Autodesk Inventor part; units mm, degrees
ref_plane "YZ Plane" through (0, 0, 0) normal (1, 0, 0) x (0, 1, 0)
ref_plane "XZ Plane" through (0, 0, 0) normal (0, 1, 0) x (-1, 0, 0)
ref_plane "XY Plane" through (0, 0, 0) normal (0, 0, 1) x (1, 0, 0)
sketch "Boceto1" plane through (0, 0, 0) normal (0, 1, 0) x (-1, 0, 0)
  line L0 (7.1, 11.7) -> (-7.1, 11.7)
  line L1 (-7.1, 11.7) -> (-7.1, -11.7)
  line L2 (-7.1, -11.7) -> (7.1, -11.7)
  line L3 (7.1, -11.7) -> (7.1, 11.7)
  line L4 (7.1, 11.7) -> (-7.1, -11.7) construction
  line L5 (-7.1, 11.7) -> (7.1, -11.7) construction
  circle A0 centre (4.1, 7.85) radius 1.45
  circle A1 centre (-4.1, 7.85) radius 1.45
  circle A2 centre (4.1, -7.85) radius 1.45
  circle A3 centre (-4.1, -7.85) radius 1.45
  point P0 (0, 0)
  dimension "d0" = 23.4
  dimension "d1" = 14.2
  dimension "d2" = 2.9
  dimension "d3" = 8.2
  dimension "d4" = 4.1
  dimension "d5" = 7.85
  dimension "d6" = 7.85
extrude "Extrusión1" add sketch "Boceto1" along normal blind 2
sketch "Boceto2" plane through (0, 2, 0) normal (0, 1, 0) x (1, 0, 0)
  line L0 (-7.1, 11.7) -> (-7.1, -11.7)
  line L1 (7.1, -3.775) -> (-7.1, -3.775)
  line L2 (-7.1, -3.775) -> (-7.1, 3.775)
  line L3 (-7.1, 3.775) -> (7.1, 3.775)
  line L4 (7.1, 3.775) -> (7.1, -3.775)
  line L5 (7.1, -3.775) -> (-7.1, 3.775) construction
  line L6 (-7.1, -3.775) -> (7.1, 3.775) construction
  point P0 (0, 0)
  point P1 (-7.1, 9.7)
  point P2 (-7.1, -9.7)
  point P3 (-7.1, -3.775)
  dimension "d10" = 7.55
extrude "Extrusión2" add sketch "Boceto2" along normal blind 2
sketch "Boceto3" plane through (0, 0, 0) normal (0, -1, 0) x (1, 0, 0)
  line L0 (-7.1, 11.7) -> (7.1, 11.7)
  line L1 (-7.1, -11.7) -> (-7.1, 11.7)
  line L2 (7.1, -11.7) -> (-7.1, -11.7)
  line L3 (7.1, 11.7) -> (7.1, -11.7)
  circle A0 centre (-4.1, 7.85) radius 1.45
  circle A1 centre (4.1, 7.85) radius 1.45
  circle A2 centre (-4.1, -7.85) radius 1.45
  circle A3 centre (4.1, -7.85) radius 1.45
  point P0 (0, 0)
extrude "Extrusión3" add sketch "Boceto3" along normal blind 14
sketch "Boceto5" plane through (0, -14, 0) normal (0, -1, 0) x (1, 0, 0)
  line L0 (7.1, -11.7) -> (7.1, 11.7)
  line L1 (-7.1, -6) -> (7.1, -6)
  line L2 (7.1, -6) -> (7.1, 6)
  line L3 (7.1, 6) -> (-7.1, 6)
  line L4 (-7.1, 6) -> (-7.1, -6)
  line L5 (-7.1, -6) -> (7.1, 6) construction
  line L6 (7.1, -6) -> (-7.1, 6) construction
  point P0 (0, 0)
  point P1 (7.1, -9.7)
  point P2 (7.1, 9.7)
  point P3 (7.1, -6)
  dimension "d16" = 12
extrude "Extrusión4" add sketch "Boceto5" along normal blind 14
sketch "Boceto7" plane through (0, -14, 0) normal (0, -1, 0) x (1, 0, 0)
  circle A0 centre (-4.1, 7.85) radius 1.45
  circle A1 centre (4.1, 7.85) radius 1.45
  circle A2 centre (4.1, -7.85) radius 1.45
  circle A3 centre (-4.1, -7.85) radius 1.45
  point P0 (0, 0)
extrude "Extrusión6" add sketch "Boceto7" against normal blind 0.5
fillet "Empalme3" radius 8 2 edges at (0, -14, 6) (0, -14, -6)
fillet "Empalme4" radius 7 2 edges at (0, -28, -6) (0, -28, 6)
fillet "Empalme5" radius 7 2 edges at (0, -14, -11.7) (0, -14, 11.7)
sketch "Boceto8" plane through (-7.1, 2, 3.775) normal (-1, 0, 0) x (0, 0, 1)
  arc A0 (-10.3083, -20.7902) -> (2.7583, -20.7902) centre (-3.775, -18.2771) ccw
  circle A1 centre (-3.775, -18.2771) radius 5.075
  point P0 (-3.775, -2)
  dimension "d28" = 10.15
extrude "Extrusión7" cut sketch "Boceto8" against normal through all
properties part number "MiddleJoint"
Source: CAD feature listing. Evaluate the final solid. Frame: model axes, mm. A direction names the side the tool comes from. Round coordinates to 2 decimals unless told otherwise and drop trailing zeros. Write each loop counter-clockwise with the first axis right and the second up, starting at its lowest first coordinate (ties: lowest second). Pieces come first, ordered by that corner, then holes. Notation, with made-up numbers: M 3.25,0 L 58.25,0 A13 ccw 58.25,21 Z; hole C 60,-38 d5. An arc over 180 degrees is marked long. One line per item, written item: value. Start each with the question number.
Item 1: Set-up query: faces 1 (the cylindrical face through (-0.1, -12.9, -11.02)), 2 (the flat face through (0, 3, 3.775)), 3 (the flat face through (0, 2, -8)), 4 (the flat face through (-4, -13.5, -8)), 5 (the cylindrical face through (0.1, -16.94, 7.54)). Return all of +Z, -Z, +X, -X, +Y, -Y with unobstructed straight access to the full face (end or side cutting, diameter ignored); none if empty.
Item 2: Section query C-C (z = -7.85). Return the cut outline in (x, y), plus the area to 3 significant figures.
Item 3: Section query A-A (y = -12.75). Return the cut outline in (x, z).
Item 4: Ray query, L1, parallel to X at y = 0.5, z = 8; L2, parallel to Z at x = 4.1, y = 0.65; L3, parallel to Z at x = -5.25, y = -4.25. Return the intervals inside material, ascending. Write a range as from..to.
Item 5: Section query D-D (y = -18). Return the cut outline in (x, z).
Item 6: Section query B-B (y = 1). Return the cut outline in (x, z), plus the area to 3 significant figures.
Item 7: Mould query, pull axis X, two halves, no side actions, for faces 6 (the flat face through (4, -13.5, -8)), 7 (the flat face through (0, -4, -11.7)), 8 (the flat face through (-7.1, -6, 0)). Classes: pulls with the +X half, pulls with the -X half, needs draft (parallel to the pull), parting line crosses it, or undercut.
Item 8: Pin query (flat end, axial travel): pin 1 (8.5 mm diameter, centred on x = 0.5, z = -6, fed in from +Y); pin 2 (2.5 mm diameter, centred on x = 4.1, z = -7.85, fed in from -Y); pin 3 (2.5 mm diameter, centred on x = -4.5, z = -7.5, fed in from +Y); pin 4 (3 mm diameter, centred on x = -3.5, z = 2, fed in from -Y). Return the tip coordinate at first contact, or that it passes through.
Result set:
1. face 1: -Z, +X, -X, -Y
1. face 2: +Z, +X, -X, +Y
1. face 3: -Z, +X, -X, +Y
1. face 4: +Y
1. face 5: +Z, +X, -X, -Y
2. outline: M -7.1,-16.55 L 7.1,-16.55 L 7.1,2 L 5.55,2 L 5.55,-13.5 L 2.65,-13.5 L 2.65,2 L -2.65,2 L -2.65,-13.5 L -5.55,-13.5 L -5.55,2 L -7.1,2 Z
2. area: 173 mm²
3. outline: M -7.1,-11.09 L 7.1,-11.09 L 7.1,-3.65 L -7.1,-3.65 Z; M -7.1,3.65 L 7.1,3.65 L 7.1,11.09 L -7.1,11.09 Z; hole C -4.1,-7.85 d2.9; hole C -4.1,7.85 d2.9; hole C 4.1,-7.85 d2.9; hole C 4.1,7.85 d2.9
4. L1: x = -7.1..-5.54, -2.66..2.66, 5.54..7.1
4. L2: z = -11.7..-9.3, -6.4..6.4, 9.3..11.7
4. L3: z = -11.7..-8.73, -6.97..6.97, 8.73..11.7
5. outline: M -7.1,-6.89 L 7.1,-6.89 L 7.1,-4.77 L -7.1,-4.77 Z; M -7.1,4.77 L 7.1,4.77 L 7.1,6.89 L -7.1,6.89 Z
6. outline: M -7.1,-11.7 L 7.1,-11.7 L 7.1,11.7 L -7.1,11.7 Z; hole C -4.1,-7.85 d2.9; hole C -4.1,7.85 d2.9; hole C 4.1,-7.85 d2.9; hole C 4.1,7.85 d2.9
6. area: 306 mm²
7. face 6: undercut
7. face 7: needs draft
7. face 8: pulls with the -X half
8. pin 1: stops at y = 4
8. pin 2: stops at y = -18.62
8. pin 3: stops at y = 2
8. pin 4: stops at y = -23.26
